Autodesk Inventor part; units mm, degrees
ref_plane "YZ Plane" through (0, 0, 0) normal (1, 0, 0) x (0, 1, 0)
ref_plane "XZ Plane" through (0, 0, 0) normal (0, 1, 0) x (-1, 0, 0)
ref_plane "XY Plane" through (0, 0, 0) normal (0, 0, 1) x (1, 0, 0)
sketch "Sketch1" plane through (0, 0, 0) normal (0, 0, 1) x (1, 0, 0)
  circle A0 centre (0, 0) radius 35
  dimension "d0" = 70
extrude "Extrusion1" add sketch "Sketch1" along normal blind 2.54
sketch "Sketch2" plane through (0, 0, 2.54) normal (0, 0, 1) x (1, 0, 0)
  line L0 (0, 0) -> (0, 34.7042) construction
  line L1 (-8.676, 28.9646) -> (8.676, 28.9646)
  line L2 (8.676, 28.9646) -> (8.676, 25.4646)
  line L3 (8.676, 25.4646) -> (-8.676, 25.4646)
  line L4 (-8.676, 25.4646) -> (-8.676, 28.9646)
  line L5 (-8.676, 28.9646) -> (8.676, 25.4646) construction
  line L6 (8.676, 28.9646) -> (-8.676, 25.4646) construction
  point P0 (0, 27.2146)
  dimension "d3" = 17.3521
  dimension "d4" = 3.5
extrude "Extrusion2" cut sketch "Sketch2" against normal blind 2.54
sketch "Sketch3" plane through (0, 0, 2.54) normal (0, 0, 1) x (1, 0, 0)
  point P0 (0, 0)
properties part number "Light Ring Mount"
CAD build for the part. Positions are in the model's coordinates, mm. A direction names the side the tool comes from. Round coordinates to 2 decimals unless told otherwise and drop trailing zeros. Order: outer loops, then holes, each group sorted by start corner. A loop starts at its lowest first (then second) coordinate and runs counter-clockwise, first axis right, second up. Notation, with made-up numbers: (-28, 80.5) - (-6, 80.5) arc R18 cw to (-6, 109.5) - close; hole circle Ø11 at (61, 65.25). An arc over 180 degrees is marked (long way). Return JSON: item names as keys, results as strings.
(1) Pin check, flat tips, straight feed: pin 1 Ø0.8 at (y, z) = (27, 1) entering from -X; pin 2 Ø10 at (x, y) = (-2, -14) entering from -Z; pin 3 Ø1.3 at (x, z) = (3, 1) entering from +Y; pin 4 Ø0.8 at (x, z) = (0, 2) entering from -Y. Stop position of each tip, or through.
Answer key:
{"pin 1": "stops at x = -22.75", "pin 2": "stops at z = 0", "pin 3": "stops at y = 34.92", "pin 4": "stops at y = -35"}
(2) Cut at C-C (y = -27.5). Give the cut face in (x, z), then the cut area to 3 significant figures.
Answer key:
{"outline": "(-21.65, 0) - (21.65, 0) - (21.65, 2.54) - (-21.65, 2.54) - close", "area": "110 mm^2"}
(3) Cut at B-B (x = 0). Give the cut face in (y, z).
Answer key:
{"outline": "(-35, 0) - (25.46, 0) - (25.46, 2.54) - (-35, 2.54) - close; (28.96, 0) - (35, 0) - (35, 2.54) - (28.96, 2.54) - close"}
(4) Cut at A-A (z = 0.4). Give the cut face in (x, y), then the cut area to 3 significant figures.
Answer key:
{"outline": "circle Ø70 at (0, 0); hole (-8.68, 25.46) - (8.68, 25.46) - (8.68, 28.96) - (-8.68, 28.96) - close", "area": "3,790 mm^2"}
(5) Tool access for faces 1 (the face through (0, 28.965, 1)), 2 (the face through (0, 0, 2.54)): list every direction of +Z, -Z, +X, -X, +Y, -Y with a clear straight run to the whole face (end or side of a thin tool).
Answer key:
{"face 1": "+Z, -Z", "face 2": "+Z, +X, -X, +Y, -Y"}
(6) Cut at D-D (x = 25.5). Give the cut face in (y, z).
Answer key:
{"outline": "(-23.97, 0) - (23.97, 0) - (23.97, 2.54) - (-23.97, 2.54) - close"}
(7) Wall check: probe 1 along Y at (x, z) = (1, 2.25); probe 2 along X at (y, z) = (-0.5, 2.4); probe 3 along X at (y, z) = (7, 1.1). Give the ranges that are in metal, low to high. Write a range as from..to.
Answer key:
{"probe 1": "y = -34.99..25.46, 28.96..34.99", "probe 2": "x = -35..35", "probe 3": "x = -34.29..34.29"}
(8) Pull direction X, two halves, no side cores. Call faces 3 (the face through (-28, 21, 1)), 4 (the face through (-8.676, 27, 1)), 5 (the face through (0, 0, 0)): +X half, -X half, draft (parallel to the pull), parting line (faces both ways), or undercut.
Answer key:
{"face 3": "parting line", "face 4": "undercut", "face 5": "draft"}
